Design review of the part built by this model. Coordinates are the model's own, in mm. A direction names the side the tool comes from. Round coordinates to 2 decimals unless told otherwise and drop trailing zeros. Order: outer loops, then holes, each group sorted by start corner. A loop starts at its lowest first (then second) coordinate and runs counter-clockwise, first axis right, second up. Notation, with made-up numbers: M -21.5,79.25 L -2.5,79.25 A30 cw -2.5,103.25 Z; hole C 15,37.5 d7. An arc over 180 degrees is marked long. Use a Markdown table: item, result. Add a question column.
(1) The part is to be moulded in two halves that separate along Y. For faces 1 (the face through (-38, -9.513, 11)), 2 (the face through (-18, -7.013, 4)), 3 (the face through (4.023, 1, 8)), say which applies: released by +Y, released by -Y, zero draft, split by the parting line, or undercut.
(2) Take a section at A-A (x = -36.5). Write out the cut boundary in (y, z).
(3) Take a section at D-D (x = -0.5). Write out the cut boundary in (y, z).
(4) Take a section at C-C (x = -5.5). Write out the cut boundary in (y, z), then the cut area to 3 significant figures.
(5) To check wall thickness, follow probe 1 along Y at (x, z) = (-16, 10); probe 2 along X at (y, z) = (-2, 6.75); probe 3 along Z at (x, y) = (-34, 9). State the ranges of each line that lie inside material, in increasing order. Write a range as from..to.
(6) Take a section at B-B (x = -18.5). Write out the cut boundary in (y, z), then the cut area to 3 significant figures.
(7) For pin 1 (1.5 mm diameter, centred on y = 11.5, z = 10, fed in from +X); pin 2 (2 mm diameter, centred on y = 0, z = 2, fed in from +X); pin 3 (3 mm diameter, centred on x = -18.5, z = 2, fed in from -Y); pin 4 (8 mm diameter, centred on x = -39, y = 0, fed in from -Z), all flat-tipped, find the tip position at first contact; note any pin that passes through.
(8) Machinability: for faces 4 (the face through (-5, 1, 0)), 5 (the face through (-38, 11.487, 11)), 6 (the face through (-18, 5, 10.5)), which of the approach directions +Z, -Z, +X, -X, +Y, -Y give a long, thin tool a straight path to every point of the face, cutting with its end or side? Answer none if there is none.
```python
from build123d import *

# Parameters (mm, degrees)
CROQUIS1_W                 = 48
CROQUIS1_H                 = 30
SALIENTE_EXTRUIR1_DEPTH    = 14
CORTAR_EXTRUIR1_DEPTH      = 36
REDONDEO1_R                = 2
REDONDEO2_R                = 7
CROQUIS3_W                 = 21.5
CROQUIS3_H                 = 18
CORTAR_EXTRUIR2_DEPTH      = 3
CORTAR_EXTRUIR3_REACH      = 50.842
CORTAR_EXTRUIR3_END_RADIUS = 18
CROQUIS5_R                 = 1
CROQUIS6_W                 = 10.8
CROQUIS6_H                 = 10.8
CORTAR_EXTRUIR4_DEPTH      = 7.5
CROQUIS7_W                 = 17
CROQUIS7_H                 = 16
CORTAR_EXTRUIR5_DEPTH      = 2
CROQUIS9_R                 = 3
SALIENTE_EXTRUIR2_DEPTH    = 30
CROQUIS10_R                = 6.25
CORTAR_EXTRUIR7_DEPTH      = 4.5
CROQUIS11_R                = 2
CORTAR_EXTRUIR8_DEPTH      = 21
CORTAR_EXTRUIR9_REACH      = 57.883
CROQUIS13_W                = 3
CROQUIS13_H                = 5
CORTAR_EXTRUIR10_DEPTH     = 3
REDONDEO3_R                = 10
CROQUIS14_R                = 2.948637221
CORTAR_EXTRUIR15_DEPTH     = 21


with BuildPart() as part:
    # Croquis1 → Saliente-Extruir1 (new body)
    with BuildSketch(Plane.XY):
        with Locations((-19.976765257, 0.987352556)):
            Rectangle(CROQUIS1_W, CROQUIS1_H)
    extrude(amount=SALIENTE_EXTRUIR1_DEPTH)

    # Croquis2 → Cortar-Extruir1 (cut)
    with BuildSketch(Plane(origin=(4.023234743, 0, 0), x_dir=(0, 0, -1), z_dir=(1, 0, 0))):
        with BuildLine():
            ThreePointArc((-14, -10.012647444), (-10.247806849, 0.987352556), (-14, 11.987352556))
            Line((-14, 11.987352556), (-14, -10.012647444))
        make_face()
    extrude(amount=-CORTAR_EXTRUIR1_DEPTH, mode=Mode.SUBTRACT)

    # Redondeo1
    redondeo1_edges = [part.edges().sort_by_distance(p)[0] for p in [
        (4.023234743, 0.987352556, 10.247806849),
    ]]
    fillet(redondeo1_edges, radius=REDONDEO1_R)

    # Redondeo2
    # the kernel refuses this fillet: 7 mm, written as the material it takes off along each edge
    with BuildSketch(Plane(origin=(-2.976765257, -7.012647444, 7), x_dir=(0, -1, 0), z_dir=(1, 0, 0))) as redondeo2_piece_1_section:
        Polygon((0, 0), (REDONDEO2_R * 1.02, 0), (REDONDEO2_R * 1.02, REDONDEO2_R * 1.02), (0, REDONDEO2_R * 1.02), align=None)
    redondeo2_piece_1 = extrude(amount=REDONDEO2_R * 1.02, mode=Mode.PRIVATE)
    redondeo2_piece_1 = redondeo2_piece_1 - Plane(origin=(-2.976765257, -7.012647444, 7), x_dir=(0, 0.7071067811865475, 0.7071067811865475), z_dir=(1, 0, 0)) * Sphere(REDONDEO2_R, mode=Mode.PRIVATE)
    add(redondeo2_piece_1, mode=Mode.SUBTRACT)
    with BuildSketch(Plane(origin=(-2.976765257, 8.987352556, 7), x_dir=(0, 0, -1), z_dir=(1, 0, 0))) as redondeo2_piece_2_section:
        Polygon((0, 0), (REDONDEO2_R * 1.02, 0), (REDONDEO2_R * 1.02, REDONDEO2_R * 1.02), (0, REDONDEO2_R * 1.02), align=None)
    redondeo2_piece_2 = extrude(amount=REDONDEO2_R * 1.02, mode=Mode.PRIVATE)
    redondeo2_piece_2 = redondeo2_piece_2 - Plane(origin=(-2.976765257, 8.987352556, 7), x_dir=(0, -0.7071067811865475, 0.7071067811865475), z_dir=(1, 0, 0)) * Sphere(REDONDEO2_R, mode=Mode.PRIVATE)
    add(redondeo2_piece_2, mode=Mode.SUBTRACT)
    with BuildSketch(Plane(origin=(-2.976765257, -14.012647444, 0), x_dir=(0, 0, 1), z_dir=(-1, 0, 0))) as redondeo2_piece_3:
        with BuildLine():
            CenterArc((REDONDEO2_R, REDONDEO2_R), REDONDEO2_R, 180, 90)
            Line((0, REDONDEO2_R), (-REDONDEO2_R * 0.02, REDONDEO2_R))
            Line((-REDONDEO2_R * 0.02, REDONDEO2_R), (-REDONDEO2_R * 0.02, -REDONDEO2_R * 0.02))
            Line((-REDONDEO2_R * 0.02, -REDONDEO2_R * 0.02), (REDONDEO2_R, -REDONDEO2_R * 0.02))
            Line((REDONDEO2_R, -REDONDEO2_R * 0.02), (REDONDEO2_R, 0))
        make_face()
    extrude(amount=58.5, mode=Mode.SUBTRACT)
    with BuildSketch(Plane(origin=(4.023234743, 8.987352556, 0), x_dir=(0, 0, 1), z_dir=(0, -1, 0))) as redondeo2_piece_4:
        with BuildLine():
            CenterArc((REDONDEO2_R, REDONDEO2_R), REDONDEO2_R, 180, 90)
            Line((0, REDONDEO2_R), (-REDONDEO2_R * 0.02, REDONDEO2_R))
            Line((-REDONDEO2_R * 0.02, REDONDEO2_R), (-REDONDEO2_R * 0.02, -REDONDEO2_R * 0.02))
            Line((-REDONDEO2_R * 0.02, -REDONDEO2_R * 0.02), (REDONDEO2_R, -REDONDEO2_R * 0.02))
            Line((REDONDEO2_R, -REDONDEO2_R * 0.02), (REDONDEO2_R, 0))
        make_face()
    extrude(amount=16, mode=Mode.SUBTRACT)
    with BuildSketch(Plane(origin=(-61.476765257, 15.987352556, 0), x_dir=(0, -1, 0), z_dir=(1, 0, 0))) as redondeo2_piece_5:
        with BuildLine():
            CenterArc((REDONDEO2_R, -REDONDEO2_R), REDONDEO2_R, 90, 90)
            Line((0, -REDONDEO2_R), (-REDONDEO2_R * 0.02, -REDONDEO2_R))
            Line((-REDONDEO2_R * 0.02, -REDONDEO2_R), (-REDONDEO2_R * 0.02, REDONDEO2_R * 0.02))
            Line((-REDONDEO2_R * 0.02, REDONDEO2_R * 0.02), (REDONDEO2_R, REDONDEO2_R * 0.02))
            Line((REDONDEO2_R, REDONDEO2_R * 0.02), (REDONDEO2_R, 0))
        make_face()
    extrude(amount=58.5, mode=Mode.SUBTRACT)
    with BuildSketch(Plane(origin=(4.023234743, 15.987352556, 7), x_dir=(0, -1, 0), z_dir=(0, 0, 1))) as redondeo2_piece_6:
        with BuildLine():
            CenterArc((REDONDEO2_R, -REDONDEO2_R), REDONDEO2_R, 90, 90)
            Line((0, -REDONDEO2_R), (-REDONDEO2_R * 0.02, -REDONDEO2_R))
            Line((-REDONDEO2_R * 0.02, -REDONDEO2_R), (-REDONDEO2_R * 0.02, REDONDEO2_R * 0.02))
            Line((-REDONDEO2_R * 0.02, REDONDEO2_R * 0.02), (REDONDEO2_R, REDONDEO2_R * 0.02))
            Line((REDONDEO2_R, REDONDEO2_R * 0.02), (REDONDEO2_R, 0))
        make_face()
    extrude(amount=24.5, mode=Mode.SUBTRACT)
    with BuildSketch(Plane(origin=(4.023234743, -14.012647444, 7), x_dir=(0, 1, 0), z_dir=(0, 0, 1))) as redondeo2_piece_7:
        with BuildLine():
            CenterArc((REDONDEO2_R, REDONDEO2_R), REDONDEO2_R, 180, 90)
            Line((0, REDONDEO2_R), (-REDONDEO2_R * 0.02, REDONDEO2_R))
            Line((-REDONDEO2_R * 0.02, REDONDEO2_R), (-REDONDEO2_R * 0.02, -REDONDEO2_R * 0.02))
            Line((-REDONDEO2_R * 0.02, -REDONDEO2_R * 0.02), (REDONDEO2_R, -REDONDEO2_R * 0.02))
            Line((REDONDEO2_R, -REDONDEO2_R * 0.02), (REDONDEO2_R, 0))
        make_face()
    extrude(amount=24.5, mode=Mode.SUBTRACT)

    # Croquis3 → Cortar-Extruir2 (cut)
    with BuildSketch(Plane(origin=(0, 0, 0), x_dir=(-1, 0, 0), z_dir=(0, 0, -1))):
        with Locations((18.226765257, 0.987352556)):
            Rectangle(CROQUIS3_W, CROQUIS3_H)
    extrude(amount=-CORTAR_EXTRUIR2_DEPTH, mode=Mode.SUBTRACT)

    # Cortar-Extruir3: up to this cylinder (the profile starts outside it)
    cortar_extruir3_end = Plane(origin=(-17.976765, 0.987352556, 28.247806849), z_dir=(1, 0, 0)) * Cylinder(CORTAR_EXTRUIR3_END_RADIUS, 138.684, mode=Mode.PRIVATE)
    # Croquis5 → Cortar-Extruir3 (cut, up to the surface)
    with BuildSketch(Plane(origin=(0, 0, 0), x_dir=(-1, 0, 0), z_dir=(0, 0, -1)), mode=Mode.PRIVATE) as cortar_extruir3_sk1:
        with Locations((17.976765257, 0.987352556)):
            Circle(CROQUIS5_R)
    cortar_extruir3_tool1 = extrude(cortar_extruir3_sk1.sketch, amount=-CORTAR_EXTRUIR3_REACH, mode=Mode.PRIVATE) - cortar_extruir3_end
    add(cortar_extruir3_tool1.solids().sort_by_distance((-17.976765, 0.987353, 0))[0], mode=Mode.SUBTRACT)

    # Croquis6 → Cortar-Extruir4 (cut)
    with BuildSketch(Plane(origin=(0, 0, 3), x_dir=(-1, 0, 0), z_dir=(0, 0, -1))):
        with Locations((17.976765257, 0.987352556)):
            Rectangle(CROQUIS6_W, CROQUIS6_H)
    extrude(amount=-CORTAR_EXTRUIR4_DEPTH, mode=Mode.SUBTRACT)

    # Croquis7 → Cortar-Extruir5 (cut)
    with BuildSketch(Plane(origin=(0, 0, 3), x_dir=(-1, 0, 0), z_dir=(0, 0, -1))):
        with Locations((17.976765257, 0.987352556)):
            Rectangle(CROQUIS7_W, CROQUIS7_H)
    extrude(amount=-CORTAR_EXTRUIR5_DEPTH, mode=Mode.SUBTRACT)

    # Croquis9 → Saliente-Extruir2 (add)
    with BuildSketch(Plane.XZ.offset(14.012647444)):
        with Locations((-38.976765257, 14)):
            Circle(CROQUIS9_R)
    extrude(amount=-SALIENTE_EXTRUIR2_DEPTH)

    # Croquis10 → Cortar-Extruir7 (cut)
    with BuildSketch(Plane(origin=(0, 15.987352556, 0), x_dir=(1, 0, 0), z_dir=(0, 1, 0))):
        with Locations((-38.976765257, -14)):
            Circle(CROQUIS10_R)
    cortar_extruir7 = extrude(amount=-CORTAR_EXTRUIR7_DEPTH, mode=Mode.SUBTRACT)

    # Simetría1: Cortar-Extruir7 across plane
    add(cortar_extruir7.mirror(Plane.ZX.offset(0.987352556)), mode=Mode.SUBTRACT)

    # Croquis11 → Cortar-Extruir8 (cut)
    with BuildSketch(Plane(origin=(0, 11.487352556, 0), x_dir=(-1, 0, 0), z_dir=(0, 1, 0))):
        with Locations(Location((38.976765257, 14, 0), (0, 0, 90))):
            Circle(CROQUIS11_R)
    extrude(amount=-CORTAR_EXTRUIR8_DEPTH, mode=Mode.SUBTRACT)

    # Cortar-Extruir9: up to this face of the body (flat: up to its plane)
    cortar_extruir9_end = Plane(part.part.faces().sort_by_distance((-19.613737998, -14.012647444, 10.301702011))[0])
    # Croquis12 → Cortar-Extruir9 (cut, up to the picked face)
    with BuildSketch(Plane(origin=(0, 15.987352556, 0), x_dir=(1, 0, 0), z_dir=(0, 1, 0)), mode=Mode.PRIVATE) as cortar_extruir9_sk1:
        Polygon((-43.976765257, -10), (-43.976765257, -14), (-41.976765257, -14), align=None)
    cortar_extruir9_tool1 = split(extrude(cortar_extruir9_sk1.sketch, amount=-CORTAR_EXTRUIR9_REACH, mode=Mode.PRIVATE), bisect_by=cortar_extruir9_end, keep=Keep.BOTH, mode=Mode.PRIVATE)
    add(cortar_extruir9_tool1.solids().sort_by(Axis((-43.310099, 15.987353, 12.666667), (0, -1, 0)))[0], mode=Mode.SUBTRACT)

    # Croquis13 → Cortar-Extruir10 (cut)
    with BuildSketch(Plane(origin=(0, 0, 0), x_dir=(-1, 0, 0), z_dir=(0, 0, -1))):
        with Locations((30.476765257, 0.987352556)):
            Rectangle(CROQUIS13_W, CROQUIS13_H)
    extrude(amount=-CORTAR_EXTRUIR10_DEPTH, mode=Mode.SUBTRACT)

    # Redondeo3
    # the kernel refuses this fillet: 10 mm, written as the material it adds along each edge
    with BuildSketch(Plane(origin=(-31.976765257, 0.987352556, 28.247806849), x_dir=(0, -0.8888591986408035, 0.45818045025036674), z_dir=(0, 0.45818045025036674, 0.8888591986408035))) as redondeo3_piece_1_section:
        with BuildLine():
            CenterArc((18 - REDONDEO3_R, REDONDEO3_R), REDONDEO3_R, 270, 90)
            Line((18 - REDONDEO3_R, 0), (18, 0))
            Line((18, 0), (18, REDONDEO3_R))
        make_face()
    redondeo3_piece_1 = revolve(axis=Axis((-31.976765257, 0.987352556, 28.247806849), (1, 0, 0)), revolution_arc=234.53951494, mode=Mode.PRIVATE)
    redondeo3_piece_1 = split(redondeo3_piece_1, bisect_by=Plane(origin=(-22.679016641, -5.92095726, 14), z_dir=(0, 0, -1)), keep=Keep.TOP, mode=Mode.PRIVATE)
    redondeo3_piece_1 = split(redondeo3_piece_1, bisect_by=Plane(origin=(-22.679016641, -5.92095726, 10.5), z_dir=(0, 0, 1)), keep=Keep.TOP, mode=Mode.PRIVATE)
    add(redondeo3_piece_1)
    with BuildSketch(Plane(origin=(-31.976765257, 0.987352556, 28.247806849), x_dir=(0, -0.8888591986408035, 0.45818045025036674), z_dir=(0, 0.45818045025036674, 0.8888591986408035))) as redondeo3_piece_2_section:
        with BuildLine():
            CenterArc((18 - REDONDEO3_R, REDONDEO3_R), REDONDEO3_R, 270, 90)
            Line((18 - REDONDEO3_R, 0), (18, 0))
            Line((18, 0), (18, REDONDEO3_R))
        make_face()
    redondeo3_piece_2 = revolve(axis=Axis((-31.976765257, 0.987352556, 28.247806849), (1, 0, 0)), revolution_arc=234.53951494, mode=Mode.PRIVATE)
    redondeo3_piece_2 = split(redondeo3_piece_2, bisect_by=Plane(origin=(-27.760529224, 0.987352545, 10.5), z_dir=(0, 0, -1)), keep=Keep.TOP, mode=Mode.PRIVATE)
    redondeo3_piece_2 = split(redondeo3_piece_2, bisect_by=Plane(origin=(-23.376765257, 0.987352545, 10.397912487), z_dir=(-1, 0, 0)), keep=Keep.TOP, mode=Mode.PRIVATE)
    add(redondeo3_piece_2)

    # Croquis14 → Cortar-Extruir15 (cut)
    with BuildSketch(Plane.ZY.offset(43.976765257)):
        with Locations(Location((4.059124212, 0.987352556, 0), (0, 0, 270))):
            Circle(CROQUIS14_R)
    extrude(amount=-CORTAR_EXTRUIR15_DEPTH, mode=Mode.SUBTRACT)


solid = part.part
```
Verdict:
| question | item | result |
|---|---|---|
| 1 | face 1 | released by -Y |
| 1 | face 2 | undercut |
| 1 | face 3 | zero draft |
| 2 | outline | M -14.01,7 A7 ccw -7.01,0 L 8.99,0 A7 ccw 15.99,7 L 15.99,8.26 L 11.49,8.26 L 11.49,15.69 L -9.51,15.69 L -9.51,8.26 L -14.01,8.26 Z; hole C 0.99,4.06 d5.9 |
| 3 | outline | M -13.56,7 A6.55 ccw -7.01,0.45 L 8.99,0.45 A6.55 ccw 15.53,7 L 15.53,14 L 11.99,14 A18 cw -10.01,14 L -13.56,14 Z |
| 4 | outline | M -14.01,7 A7 ccw -7.01,0 L 8.99,0 A7 ccw 15.99,7 L 15.99,14 L 11.99,14 A18 cw -10.01,14 L -14.01,14 Z |
| 4 | area | 343 mm^2 |
| 5 | probe 1 | y = -14.01..-4.41, 6.39..15.99 |
| 5 | probe 2 | x = -43.98..-23.38, -12.58..4.02 |
| 5 | probe 3 | z = 0..14 |
| 6 | outline | M -14.01,7 A7 ccw -8.01,0.07 L -8.01,3 L -7.01,3 L -7.01,5 L -4.41,5 L -4.41,10.5 L -2.02,10.5 A18 cw -10.01,14 L -14.01,14 Z; M 3.99,10.5 L 6.39,10.5 L 6.39,5 L 8.99,5 L 8.99,3 L 9.99,3 L 9.99,0.07 A7 ccw 15.99,7 L 15.99,14 L 11.99,14 A18 cw Z |
| 6 | area | 198 mm^2 |
| 7 | pin 1 | stops at x = 3.8 |
| 7 | pin 2 | stops at x = 2.77 |
| 7 | pin 3 | stops at y = -13.07 |
| 7 | pin 4 | stops at z = 0 |
| 8 | face 4 | -Z, +X, -X, +Y, -Y |
| 8 | face 5 | +Z, +Y |
| 8 | face 6 | -Z |
